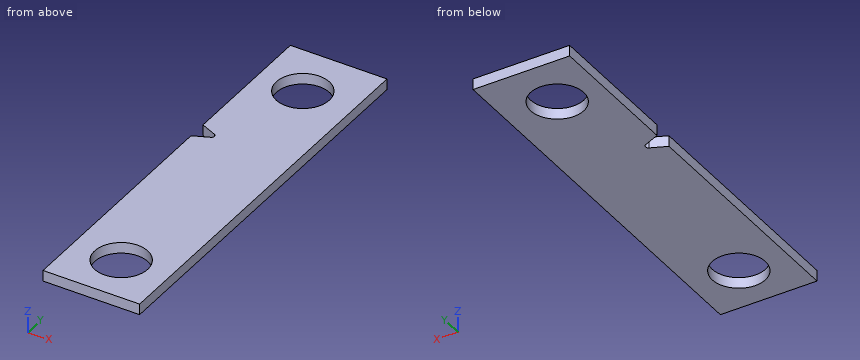
from build123d import *

# Parameters (mm, degrees)
SKETCH1_W           = 42.5
SKETCH1_H           = 40
BOSS_EXTRUDE1_DEPTH = 2.25
SKETCH3_R           = 11
CUT_EXTRUDE2_DEPTH  = 5
SKETCH4_W           = 42.5
SKETCH4_H           = 4.5
BOSS_EXTRUDE2_DEPTH = 15
SKETCH8_W           = 2.5
SKETCH8_H           = 55
CUT_EXTRUDE4_DEPTH  = 10
SKETCH9_W           = 40
SKETCH9_H           = 4.5
BOSS_EXTRUDE3_DEPTH = 110.599864081
SKETCH11_R          = 11
CUT_EXTRUDE5_DEPTH  = 100
CUT_EXTRUDE6_DEPTH  = 100


with BuildPart() as part:
    # Sketch1 → Boss-Extrude1 (new, symmetric)
    with BuildSketch(Plane.XY):
        Rectangle(SKETCH1_W, SKETCH1_H)
    extrude(amount=BOSS_EXTRUDE1_DEPTH, both=True)

    # Sketch3 → Cut-Extrude2 (cut, symmetric)
    with BuildSketch(Plane.XY.offset(2.25)):
        with Locations((1.25, 0)):
            Circle(SKETCH3_R)
    extrude(amount=CUT_EXTRUDE2_DEPTH, both=True, mode=Mode.SUBTRACT)

    # Sketch4 → Boss-Extrude2 (add)
    with BuildSketch(Plane(origin=(0, 20, 0), x_dir=(1, 0, 0), z_dir=(0, 1, 0))):
        Rectangle(SKETCH4_W, SKETCH4_H)
    extrude(amount=BOSS_EXTRUDE2_DEPTH)

    # Sketch8 → Cut-Extrude4 (cut)
    with BuildSketch(Plane.XY.offset(2.25)):
        with Locations((-20, 7.5)):
            Rectangle(SKETCH8_W, SKETCH8_H)
    extrude(amount=-CUT_EXTRUDE4_DEPTH, mode=Mode.SUBTRACT)

    # Sketch9 → Boss-Extrude3 (add)
    with BuildSketch(Plane(origin=(0, 35, 0), x_dir=(1, 0, 0), z_dir=(0, 1, 0))):
        with Locations((1.25, 0)):
            Rectangle(SKETCH9_W, SKETCH9_H)
    extrude(amount=BOSS_EXTRUDE3_DEPTH)

    # Sketch11 → Cut-Extrude5 (cut)
    with BuildSketch(Plane(origin=(0, 0, -2.25), x_dir=(-1, 0, 0), z_dir=(0, 0, -1))):
        with Locations((0, 123.599864081)):
            Circle(SKETCH11_R)
    extrude(amount=-CUT_EXTRUDE5_DEPTH, mode=Mode.SUBTRACT)

    # Sketch12 → Cut-Extrude6 (cut)
    with BuildSketch(Plane(origin=(0, 0, -2.25), x_dir=(-1, 0, 0), z_dir=(0, 0, -1))):
        with BuildLine():
            Line((18.75, 79.099864081), (18.75, 87.099864081))
            Line((18.75, 87.099864081), (12.247409908, 84.244374107))
            ThreePointArc((12.247409908, 84.244374107), (11.5, 83.099864066), (12.247409936, 81.955354043))
            Line((12.247409936, 81.955354043), (18.75, 79.099864081))
        make_face()
    extrude(amount=-CUT_EXTRUDE6_DEPTH, mode=Mode.SUBTRACT)


solid = part.part
Build history of the part. All positions in model axes, mm. Give positions to 0.01 mm unless a question says otherwise; leave off trailing zeros. Order: outer loops, then holes, each group sorted by start corner. A loop starts at its lowest first (then second) coordinate and runs counter-clockwise, first axis right, second up. Notation, with made-up numbers: M 24.5,40.5 L 54.5,40.5 A31 ccw 54.5,68.5 Z; hole C -29.5,-6.5 d9. An arc over 180 degrees is marked long. Put each result on its own line as item: value.
Item 1: Cut at B-B on x = 1.25. Write the cut outline in (y, z).
Results are:
outline: M -20,-2.25 L -11,-2.25 L -11,2.25 L -20,2.25 Z; M 11,-2.25 L 112.67,-2.25 L 112.67,2.25 L 11,2.25 Z; M 134.53,-2.25 L 145.6,-2.25 L 145.6,2.25 L 134.53,2.25 Z
Item 2: Cut at A-A on y = 0. Write the cut outline in (x, z).
Results are:
outline: M -18.75,-2.25 L -9.75,-2.25 L -9.75,2.25 L -18.75,2.25 Z; M 12.25,-2.25 L 21.25,-2.25 L 21.25,2.25 L 12.25,2.25 Z
Item 3: Cut at D-D on y = 121. Write the cut outline in (x, z), then the cut area to 3 significant figures.
Results are:
outline: M -18.75,-2.25 L -10.69,-2.25 L -10.69,2.25 L -18.75,2.25 Z; M 10.69,-2.25 L 21.25,-2.25 L 21.25,2.25 L 10.69,2.25 Z
area: 83.8 mm2
Item 4: Drop a flat-ended pin along its axis: pin 1 Ø2 at (y, z) = (82, 0.5) entering from -X. Give the stop position or say it passes through.
Results are:
pin 1: x = -14.42
Item 5: Wall check: probe 1 along Y at (x, z) = (0.5, -0.6); probe 2 along Y at (x, z) = (1.25, -1.15); probe 3 along X at (y, z) = (123.5, 0.65). Give the ranges that are in metal, low to high.
Results are:
probe 1: -20 to -10.97, 10.97 to 112.61, 134.59 to 145.6
probe 2: -20 to -11, 11 to 112.67, 134.53 to 145.6
probe 3: -18.75 to -11, 11 to 21.25
Item 6: Cut at C-C on z = -0.3. Write the cut outline in (x, y).
Results are:
outline: M -18.75,-20 L 21.25,-20 L 21.25,145.6 L -18.75,145.6 L -18.75,87.1 L -12.25,84.24 A1.25 cw -12.25,81.96 L -18.75,79.1 Z; hole C 0,123.6 d22; hole C 1.25,0 d22
